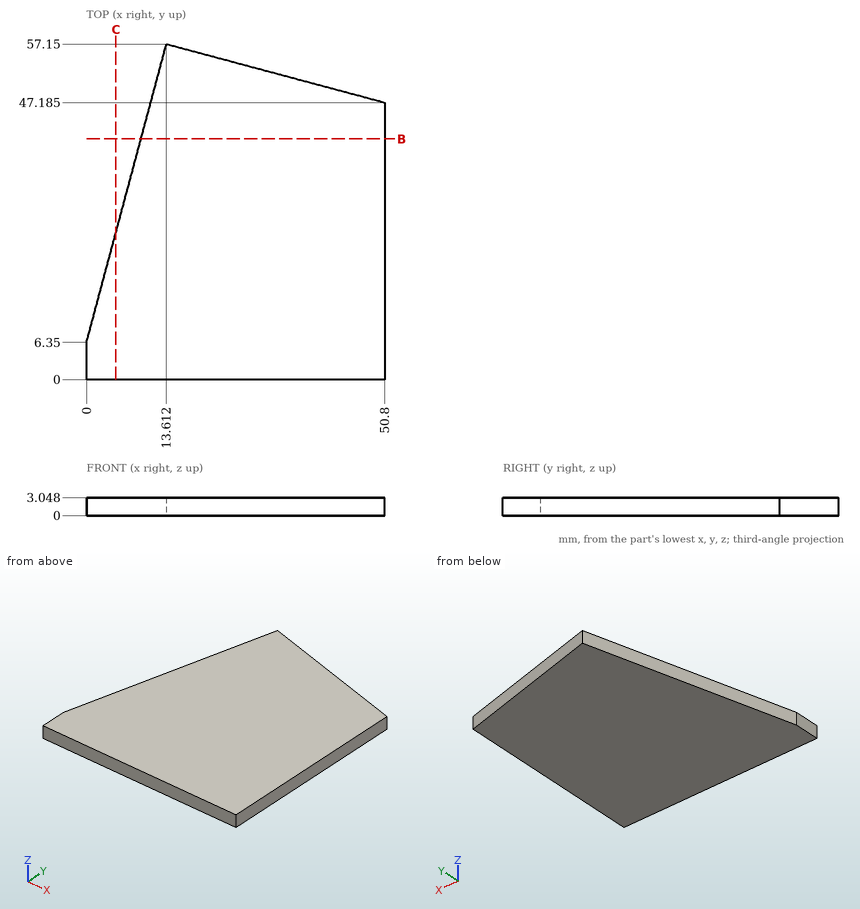
Answer from the drawing. Dimensions are ordinates in mm from the lowest x, y and z of the part. Round coordinates to 2 decimals unless told otherwise and drop trailing zeros. Write each loop counter-clockwise with the first axis right and the second up, starting at its lowest first coordinate (ties: lowest second). Pieces come first, ordered by that corner, then holes. Notation, with made-up numbers: M 68,-14 L 75,-14 A11 ccw 75,-6 Z; hole C -21.5,28 d9. An arc over 180 degrees is marked long. Write each question's results on one line, items separated by ' | '. Start each with the question number.
Item 1: Find section C-C on x = 5. Write down the section's boundary in (y, z).
Item 2: Straight lines are drawn through the part: probe 1 along Y at (x, z) = (23, 0.35) (1 decimal); probe 2 along X at (y, z) = (6.5, 2.55); probe 3 along Y at (x, z) = (32, 2.7). For each, find the intervals that lie inside material, in ascending order.
Item 3: Find section B-B on y = 41. Write down the section's boundary in (x, z) (1 decimal).
Answer block:
1) outline: M 0,0 L 25.01,0 L 25.01,3.05 L 0,3.05 Z
2) probe 1: y = 0 to 54.6 | probe 2: x = 0.04 to 50.8 | probe 3: y = 0 to 52.22
3) outline: M 9.3,0 L 50.8,0 L 50.8,3 L 9.3,3 Z
